Autodesk Inventor part; units mm, degrees
ref_plane "YZ Plane" through (0, 0, 0) normal (1, 0, 0) x (0, 1, 0)
ref_plane "XZ Plane" through (0, 0, 0) normal (0, 1, 0) x (-1, 0, 0)
ref_plane "XY Plane" through (0, 0, 0) normal (0, 0, 1) x (1, 0, 0)
sketch "Esboço1" plane through (0, 0, 0) normal (0, 1, 0) x (-1, 0, 0)
  line L0 (0, 0) -> (252, 0)
  line L1 (252, 0) -> (252, -158)
  line L2 (252, -158) -> (0, -158)
  line L3 (0, -158) -> (0, 0)
  dimension "d0" = 252
  dimension "d1" = 158
extrude "Extrusão1" add sketch "Esboço1" along normal blind 4
fillet "Arredondamento1" radius 2 4 edges at (0, 2, 0) (0, 2, -158) (-252, 2, 0) (-252, 2, -158)
sketch "Esboço2" plane through (0, 4, 0) normal (0, 1, 0) x (1, 0, 0)
  circle A0 centre (-244, 150) radius 3.35
  circle A1 centre (-244, 8) radius 3.35
  circle A2 centre (-8, 150) radius 3.35
  circle A3 centre (-8, 8) radius 3.35
  line L0 (-252, 156) -> (-252, 2)
  line L1 (-2, 158) -> (-250, 158)
  line L2 (-250, 0) -> (-2, 0)
  line L3 (0, 2) -> (0, 156)
  point P0 (0, 0)
  dimension "d5" = 6.7
  dimension "d6" = 6.7
  dimension "d7" = 6.7
  dimension "d8" = 6.7
  dimension "d9" = 8
  dimension "d10" = 8
  dimension "d11" = 8
  dimension "d12" = 8
  dimension "d13" = 8
  dimension "d14" = 8
  dimension "d15" = 8
  dimension "d16" = 8
extrude "Extrusão2" cut sketch "Esboço2" against normal blind 10
sketch "Esboço3" plane through (0, 0, 0) normal (0, -1, 0) x (1, 0, 0)
  line L0 (-14.2, -140.75) -> (-87.5029, -140.75)
  arc A0 (-89.0029, -139.25) -> (-87.5029, -140.75) centre (-87.5029, -139.25) ccw
  line L1 (-89.0029, -130.5) -> (-89.0029, -139.25)
  line L2 (-89.0029, -130.5) -> (-89.0029, -10.5)
  line L3 (-89.0029, -1.75) -> (-89.0029, -10.5)
  arc A1 (-87.5029, -0.25) -> (-89.0029, -1.75) centre (-87.5029, -1.75) ccw
  line L4 (-87.5029, -0.25) -> (-14.2, -0.25)
  line L5 (-14.2, -140.75) -> (-14.2, -0.25)
  circle A2 centre (-31, -21) radius 2
  circle A3 centre (-31, -21) radius 4
  circle A4 centre (-41, -31) radius 2
  circle A5 centre (-31, -21) radius 2
  circle A6 centre (-31, -121) radius 4.5
  circle A7 centre (-82, -111) radius 2
  circle A8 centre (-41, -111) radius 2
  circle A9 centre (-72, -121) radius 2
  circle A10 centre (-72, -121) radius 4.5
  circle A11 centre (-41, -31) radius 2
  circle A12 centre (-82, -31) radius 2
  circle A13 centre (-72, -21) radius 2
  circle A14 centre (-72, -21) radius 4.5
  point P0 (0, 0)
extrude "Extrusão3" cut sketch "Esboço3" against normal blind 10 contours A4 | A7 | A8 | A12
sketch "Esboço4" plane through (0, 4, 0) normal (0, 1, 0) x (1, 0, 0)
  circle A0 centre (-216, 148) radius 2
  circle A1 centre (-108, 137) radius 2
  circle A2 centre (-119, 149) radius 2
  circle A3 centre (-228, 137) radius 2
  circle A4 centre (-227, 21) radius 2
  circle A5 centre (-216, 9) radius 2
  circle A6 centre (-108, 21) radius 2
  circle A7 centre (-119, 9) radius 2
  point P0 (0, 0)
  point P1 (-122.4, 150.963)
extrude "Extrusão4" cut sketch "Esboço4" against normal blind 10
sketch "Esboço5" plane through (0, 4, 0) normal (0, 1, 0) x (1, 0, 0)
  circle A0 centre (-178.16, 71.72) radius 1.5
  circle A1 centre (-178.1, 43.84) radius 1.5
  circle A2 centre (-228.96, 28.5) radius 1.5
  circle A3 centre (-230.23, 76.8) radius 1.5
  point P0 (0, 0)
extrude "Extrusão5" cut sketch "Esboço5" against normal blind 10
equation "\"d8\" = d6"
equation "\"d10\" = d12"
equation "\"d11\" = d10"
equation "\"d12\" = d9"
equation "\"d13\" = d12"
equation "\"d14\" = d13"
equation "\"d15\" = d13"
equation "\"d16\" = d15"
properties part number "Base"
The listing builds one solid part. Answer for the finished solid, in the listing's coordinates (mm). Give positions to 0.01 mm unless a question says otherwise; leave off trailing zeros. Return JSON: item names as keys, results as strings. Group by question number.
1. Straight lines are drawn through the part: line 1 (Z direction, x = -82, y = 1.7); line 2 (X direction, y = 3.1, z = -28.5); line 3 (X direction, y = 1.9, z = -71.72). For each, find the intervals that lie inside material, in ascending order. Write a range as [from, to].
2. Determine the mould class of faces 1 (the cylindrical face through (-247.347, 2.028, -8.147)), 2 (the flat face through (-124, 4, -78)), 3 (the cylindrical face through (-8.73, 2.03, -146.73)) for opening direction Z: pulls with the +Z half, pulls with the -Z half, needs draft (parallel to the pull), parting line crosses it, or undercut.
3. Given pin 1 Ø2.5 at (x, z) = (-108, -21) entering from +Y, flat-ended and moving along its own axis, determine where the tip first touches the part or whether it passes through.
Verdict:
{
 "1": {"line 1": "z = [-158, -113], [-109, -33], [-29, 0]", "line 2": "x = [-252, -230.46], [-227.46, 0]", "line 3": "x = [-252, -179.66], [-176.66, 0]"},
 "2": {"face 1": "undercut", "face 2": "needs draft", "face 3": "undercut"},
 "3": {"pin 1": "passes through"}
}
